Work out the finished part from the listing and answer in its coordinate system (mm). Face numbers are marked on the shaded views. A direction names the side the tool comes from. Give positions to 0.01 mm unless a question says otherwise; leave off trailing zeros. Write each loop counter-clockwise with the first axis right and the second up, starting at its lowest first coordinate (ties: lowest second). Pieces come first, ordered by that corner, then holes. Notation, with made-up numbers: (-20, -18) - (16, -18) arc R15 ccw to (16, -6) - close; hole circle Ø11 at (-6, -2.75). An arc over 180 degrees is marked (long way). Write each question's results on one line, items separated by ' | '. Start each with the question number.
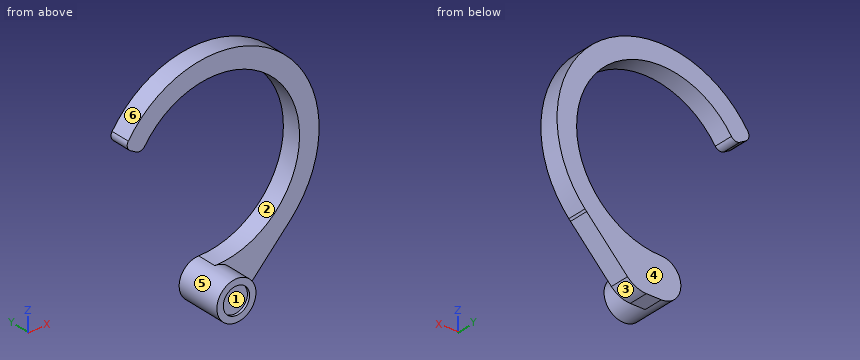
from build123d import *

# Parameters (mm, degrees)
EXTRUDE_4_DEPTH     = 15
EXTRUDE_START       = 20
SKETCH_4_R          = 15
EXTRUDE_5_DEPTH     = 20
SKETCH_5_R          = 10.1
CUT_EXTRUDE_1_DEPTH = 2


with BuildPart() as part:
    # ｽｹｯﾁ2 → ﾎﾞｽ - 押し出し4 (new body)
    with BuildSketch(Plane(origin=(0, 0, 0), x_dir=(1, 0, 0), z_dir=(0, 1, 0))):
        with BuildLine():
            ThreePointArc((-53.82643789, -36.437818048), (-56.846261527, -34.367935813), (-60.466933112, -34.910600109))
            Line((-60.466933112, -34.910600109), (-64.807406984, -37.416573868))
            ThreePointArc((-64.807406984, -37.416573868), (-67.177509772, -40.614402853), (-66.461234116, -44.529814279))
            ThreePointArc((-66.461234116, -44.529814279), (49.665387485, -62.716419588), (58.57572973, 54.487465409))
            Line((58.57572973, 54.487465409), (57.289371136, 55.838409315))
            Line((57.289371136, 55.838409315), (25.911523347, 88.791671712))
            ThreePointArc((25.911523347, 88.791671712), (19.306695871, 93.382511176), (11.427401304, 95))
            Line((11.427401304, 95), (0, 95))
            ThreePointArc((0, 95), (-15, 80), (0, 65))
            ThreePointArc((0, 65), (57.41714976, -30.467538684), (-53.82643789, -36.437818048))
        make_face()
    extrude(amount=EXTRUDE_4_DEPTH)

    # ｽｹｯﾁ4 → ﾎﾞｽ - 押し出し5 (add)
    with BuildSketch(Plane.XZ.offset(EXTRUDE_START)):
        with Locations(Location((0, -80, 0), (0, 0, 270))):
            Circle(SKETCH_4_R)
    extrude(amount=-EXTRUDE_5_DEPTH)

    # ｽｹｯﾁ5 → ｶｯﾄ - 押し出し1 (cut)
    with BuildSketch(Plane(origin=(0, -20, 0), x_dir=(-1, 0, 0), z_dir=(0, -1, 0))):
        with Locations(Location((0, 80, 0), (0, 0, 90))):
            Circle(SKETCH_5_R)
    extrude(amount=-CUT_EXTRUDE_1_DEPTH, mode=Mode.SUBTRACT)


solid = part.part
Q1. A tool of negligible diameter and unlimited length cuts with its end or side. For the marked faces 5 and 6, from which of +Z, -Z, +X, -X, +Y, -Y can it reach the whole face along a straight path? Write none if from no direction.
Q2. The mould has two halves that part along X. Classify the marked faces 1, 2, 3 and 4: pulls with the +X half, pulls with the -X half, needs draft (parallel to the pull), parting line crosses it, or undercut.
Q3. A cutting plane is placed at D-D, the plane y = -15. Write down the section's boundary in (x, z), and give its area (3 significant figures).
Q4. A cutting plane is placed at B-B, the plane x = 22. Write down the section's boundary in (y, z).
Q5. A cutting plane is placed at C-C, the plane z = -80. Write down the section's boundary in (x, y).
Q6. A cutting plane is placed at A-A, the plane y = 11. Write down the section's boundary in (x, z), and give its area (3 significant figures).
Q7. Given pin 1 (1 mm diameter, centred on x = 32.5, z = 59.5, fed in from -Y); pin 2 (6 mm diameter, centred on y = 5.5, z = -53, fed in from +X); pin 3 (4 mm diameter, centred on x = -20.5, y = 6, fed in from -Z); pin 4 (6 mm diameter, centred on y = -5.5, z = 5, fed in from +X), each flat-ended and moving along its own axis, determine where each tip first touches the part or whether it passes through.
Q8. Consider L1, parallel to Z at x = 0, y = 3; L2, parallel to Y at x = -44.5, z = 52.5; L3, parallel to X at y = -18.75, z = -80. Determine where each line is inside the solid, lowest interval first.
Result:
1) face 5: -Y | face 6: +Y, -Y
2) face 1: undercut | face 2: undercut | face 3: pulls with the +X half | face 4: needs draft
3) outline: circle Ø30 at (0, -80) | area: 707 mm2
4) outline: (0, -91.98) - (15, -91.98) - (15, -61.16) - (0, -61.16) - close; (0, 61.16) - (15, 61.16) - (15, 76.92) - (0, 76.92) - close
5) outline: (-15, -20) - (-10.1, -20) - (-10.1, -18) - (10.1, -18) - (10.1, -20) - (15, -20) - (15, 0) - (34.28, 0) - (34.28, 15) - (-15, 15) - close
6) outline: (-66.46, 44.53) arc R5 ccw to (-64.81, 37.42) - (-60.47, 34.91) arc R5 ccw to (-53.83, 36.44) arc R65 cw (long way) to (0, -65) arc R15 ccw to (0, -95) - (11.43, -95) arc R20 ccw to (25.91, -88.79) - (58.58, -54.49) arc R80 ccw (long way) to start | area: 5,450 mm2
7) pin 1: stops at y = 0 | pin 2: stops at x = 62.45 | pin 3: stops at z = 60.98 | pin 4: passes through
8) L1: z = -95 to -65, 65 to 80 | L2: y = 0 to 15 | L3: x = -15 to -10.1, 10.1 to 15
